Model file for the job. Use its own axes, mm. A direction names the side the tool comes from. Give positions to 0.01 mm unless a question says otherwise; leave off trailing zeros. Write each loop counter-clockwise with the first axis right and the second up, starting at its lowest first coordinate (ties: lowest second). Pieces come first, ordered by that corner, then holes. Notation, with made-up numbers: (64, 14.5) - (92, 14.5) arc R23 cw to (92, 34.5) - close; hole circle Ø9 at (-17.5, 86.25). An arc over 180 degrees is marked (long way). Use CSV: the item, a comma, the result in double quotes.
from build123d import *

# Parameters (mm, degrees)
EXTRUDE_THIN1_DEPTH = 40
FILLET1_R           = 10
FILLET2_R           = 10
FILLET3_R           = 10
FILLET4_R           = 10


with BuildPart() as part:
    # Sketch1 → Extrude-Thin1 (new body)
    with BuildSketch(Plane.XY):
        with BuildLine():
            Line((50, 0), (8.078800395, 0))
            ThreePointArc((8.078800395, 0), (1.794545597, 2.221302061), (-1.697863575, 7.898371675))
            Line((-1.697863575, 7.898371675), (-12.609769953, 58.65998382))
            Line((-12.609769953, 58.65998382), (-2.833105983, 60.761612145))
            Line((-2.833105983, 60.761612145), (8.078800395, 10))
            Line((8.078800395, 10), (50, 10))
            Line((50, 10), (50, 0))
        make_face()
    extrude(amount=EXTRUDE_THIN1_DEPTH)

    # Fillet1
    fillet1_edges = [part.edges().sort_by_distance(p)[0] for p in [
        (-7.721437968, 59.710797982, 40),
    ]]
    fillet(fillet1_edges, radius=FILLET1_R)

    # Fillet2
    fillet2_edges = [part.edges().sort_by_distance(p)[0] for p in [
        (50, 5, 40),
    ]]
    fillet(fillet2_edges, radius=FILLET2_R)

    # Fillet3
    fillet3_edges = [part.edges().sort_by_distance(p)[0] for p in [
        (50, 5, 0),
    ]]
    fillet(fillet3_edges, radius=FILLET3_R)

    # Fillet4
    fillet4_edges = [part.edges().sort_by_distance(p)[0] for p in [
        (-7.721437968, 59.710797982, 0),
    ]]
    fillet(fillet4_edges, radius=FILLET4_R)


solid = part.part
(1) Saw through at B-B, the plane y = 9. List the corners of the cut face in (x, z), then the cut area to 3 significant figures.
Checked values:
outline,"(-1.93, 0) - (40, 0) arc R10 ccw to (50, 10) - (50, 30) arc R10 ccw to (40, 40) - (-1.93, 40) - close"
area,"2,030 mm^2"
(2) Wall check: probe 1 along Y at (x, z) = (16, 22.5); probe 2 along X at (y, z) = (52.5, 36.5); probe 3 along X at (y, z) = (38.5, 29). Give the ranges that are in metal, low to high. Write a range as [from, to].
Checked values:
probe 1,"y = [0, 10]"
probe 2,"x = [-11.29, -1.06]"
probe 3,"x = [-8.28, 1.95]"
(3) Saw through at A-A, the plane z = 25.5. List the corners of the cut face in (x, y), then the cut area to 3 significant figures.
Checked values:
outline,"(-12.61, 58.66) - (-1.7, 7.9) arc R10 ccw to (8.08, 0) - (50, 0) - (50, 10) - (8.08, 10) - (-2.83, 60.76) - close"
area,"1,010 mm^2"
(4) Saw through at C-C, the plane x = 19.5. List the corners of the cut face in (y, z), then the cut area to 3 significant figures.
Checked values:
outline,"(0, 0) - (10, 0) - (10, 40) - (0, 40) - close"
area,"400 mm^2"
(5) 3-axis set-ups, long thin cutter, end or side, ignore diameter. For faces 1 (the face through (-7.077, 32.924, 19.72)), 2 (the face through (29, 10, 20)): which of +Z, -Z, +X, -X, +Y, -Y reach the whole face in a straight line?
Checked values:
face 1,"+Z, -Z, -X, -Y"
face 2,"+Z, -Z, +X, +Y"
(6) Flat gauge pins, fed straight in: P1, Ø3, axis at x = 22, z = 15, coming from the +Y side; P2, Ø2, axis at y = 52, z = 29.5, coming from the +X side. Where does each tip first touch, or does it go through?
Checked values:
P1,"stops at y = 10"
P2,"stops at x = -0.73"
(7) Saw through at D-D, the plane z = 4.5. List the corners of the cut face in (x, y).
Checked values:
outline,"(-12.26, 57.05) - (-1.7, 7.9) arc R10 ccw to (8.08, 0) - (48.35, 0) - (48.35, 10) - (8.08, 10) - (-2.49, 59.15) - close"
